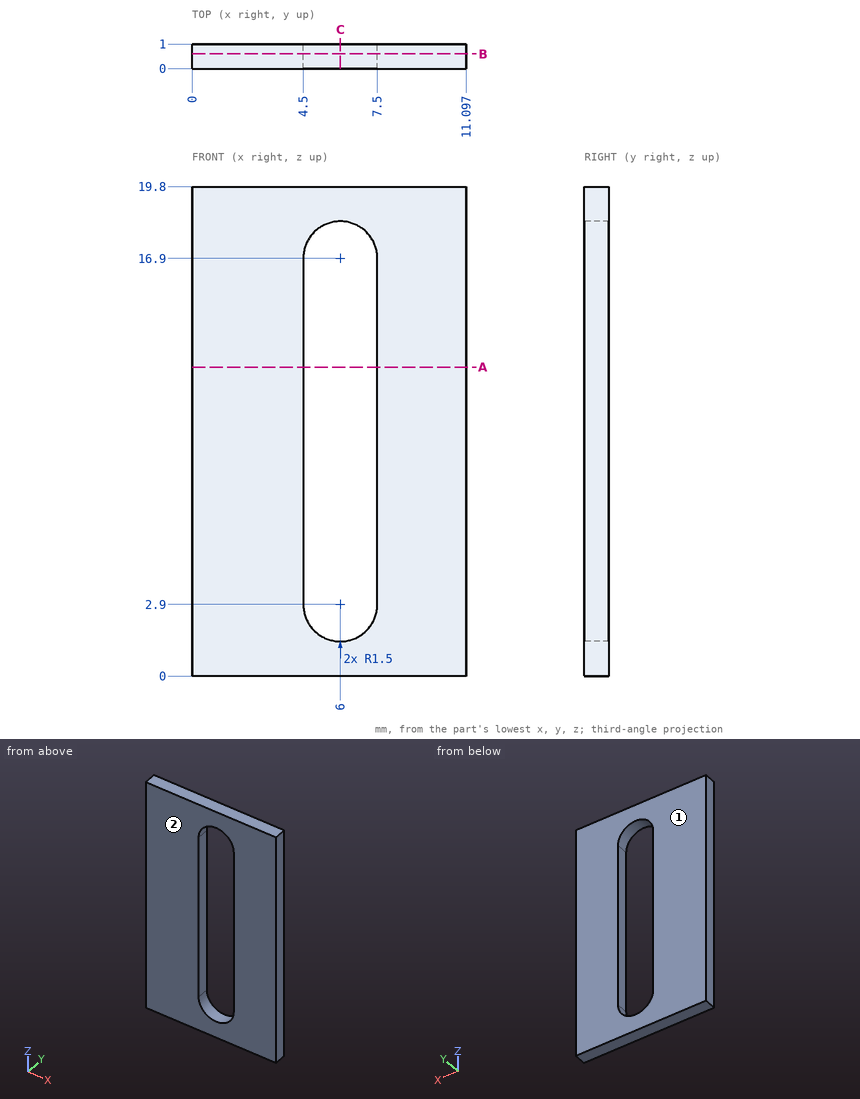
Here's the drawing with two shaded views (mm, measured from the low corner). I have some questions. Give positions to 0.01 mm unless a question says otherwise; leave off trailing zeros. Loops run counter-clockwise (first coordinate to the right, second up) from the corner with the lowest first, then second, coordinate; pieces in that order, holes last. Notation, with made-up numbers: M 38,66 L 88,66 A11 cw 88,87 Z; hole C 56.25,25 d1. An arc over 180 degrees is marked long. One line per item, written item: value.
(1) Suppose I cut it at B-B on y = 0.6. List the corners of the cut face in (x, z) for me, plus the area to 3 significant figures.
Returned:
outline: M 0,0 L 11.1,0 L 11.1,19.8 L 0,19.8 Z; hole M 4.5,2.9 A1.5 ccw 7.5,2.9 L 7.5,16.9 A1.5 ccw 4.5,16.9 Z
area: 171 mm^2
(2) Suppose I cut it at C-C on x = 6. List the corners of the cut face in (y, z) for me, plus the area to 3 significant figures.
Returned:
outline: M 0,0 L 1,0 L 1,1.4 L 0,1.4 Z; M 0,18.4 L 1,18.4 L 1,19.8 L 0,19.8 Z
area: 2.80 mm^2
(3) We'd pull the mould along Y, two halves only. Please class the marked faces 1 and 2: released by +Y, released by -Y, zero draft, split by the parting line, or undercut.
Returned:
face 1: released by +Y
face 2: released by -Y
(4) Suppose I cut it at A-A on z = 12.5. List the corners of the cut face in (x, y) for me.
Returned:
outline: M 0,0 L 4.5,0 L 4.5,1 L 0,1 Z; M 7.5,0 L 11.1,0 L 11.1,1 L 7.5,1 Z
(5) I need wall thicknesses on line 1 (X direction, y = 0.7, z = 11.75); line 2 (Z direction, x = 7, y = 0.8); line 3 (Z direction, x = 6.25, y = 0.6). Which ranges of each line are inside material? Lowest first, please.
Returned:
line 1: 0 to 4.5, 7.5 to 11.1
line 2: 0 to 1.78, 18.02 to 19.8
line 3: 0 to 1.42, 18.38 to 19.8
